Answer from the drawing. Dimensions are ordinates in mm from the lowest x, y and z of the part. Give positions to 0.01 mm unless a question says otherwise; leave off trailing zeros. Write each loop counter-clockwise with the first axis right and the second up, starting at its lowest first coordinate (ties: lowest second). Pieces come first, ordered by that corner, then holes.
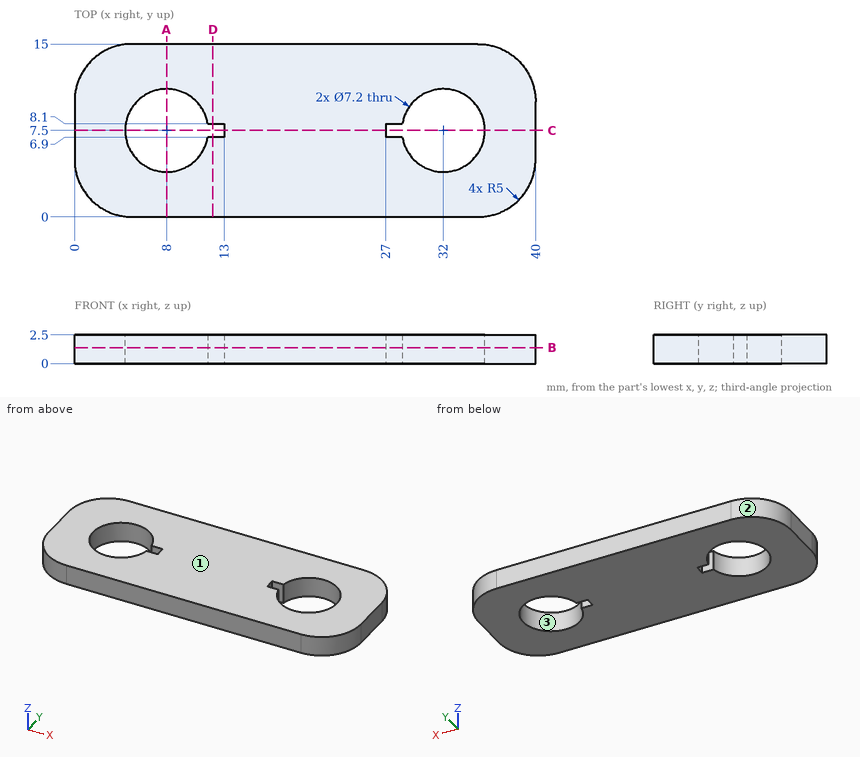
Item 1: A cutting plane is placed at A-A, the plane x = 8. Give the vertices of the cut face in (y, z), plus the area to 3 significant figures.
Conclusion:
outline: (0, 0) - (3.9, 0) - (3.9, 2.5) - (0, 2.5) - close; (11.1, 0) - (15, 0) - (15, 2.5) - (11.1, 2.5) - close
area: 19.5 mm2
Item 2: A cutting plane is placed at B-B, the plane z = 1.4. Give the vertices of the cut face in (x, y).
Conclusion:
outline: (0, 5) arc R5 ccw to (5, 0) - (35, 0) arc R5 ccw to (40, 5) - (40, 10) arc R5 ccw to (35, 15) - (5, 15) arc R5 ccw to (0, 10) - close; hole (11.55, 6.9) - (13, 6.9) - (13, 8.1) - (11.55, 8.1) arc R3.6 ccw (long way) to start; hole (27, 6.9) - (28.45, 6.9) arc R3.6 ccw (long way) to (28.45, 8.1) - (27, 8.1) - close
Item 3: A cutting plane is placed at C-C, the plane y = 7.5. Give the vertices of the cut face in (x, z).
Conclusion:
outline: (0, 0) - (4.4, 0) - (4.4, 2.5) - (0, 2.5) - close; (13, 0) - (27, 0) - (27, 2.5) - (13, 2.5) - close; (35.6, 0) - (40, 0) - (40, 2.5) - (35.6, 2.5) - close
Item 4: Determine the mould class of the marked faces 1, 2 and 3 for opening direction X: pulls with the +X half, pulls with the -X half, needs draft (parallel to the pull), parting line crosses it, or undercut.
Conclusion:
face 1: needs draft
face 2: pulls with the -X half
face 3: undercut
Item 5: Each of these flat-tipped pins is pushed along its axis until it touches: P1, Ø1.5, axis at y = 11, z = 1, coming from the +X side; P2, Ø5, axis at x = 20, y = 12, coming from the -Z side. Where does it stop, or does it pass through?
Conclusion:
P1: stops at x = 39.99
P2: stops at z = 0
Item 6: A cutting plane is placed at D-D, the plane x = 12. Give the vertices of the cut face in (y, z), plus the area to 3 significant figures.
Conclusion:
outline: (0, 0) - (6.9, 0) - (6.9, 2.5) - (0, 2.5) - close; (8.1, 0) - (15, 0) - (15, 2.5) - (8.1, 2.5) - close
area: 34.5 mm2
Item 7: Consider probe 1 along X at (y, z) = (7.5, 0.6); probe 2 along Y at (x, z) = (32, 0.65); probe 3 along X at (y, z) = (6.75, 2.2). Determine where each line is inside the solid, lowest interval first.
Conclusion:
probe 1: x = 0 to 4.4, 13 to 27, 35.6 to 40
probe 2: y = 0 to 3.9, 11.1 to 15
probe 3: x = 0 to 4.48, 11.52 to 28.48, 35.52 to 40
